Geometry: final body of the model. Coordinates: model frame, mm. A direction names the side the tool comes from. Give positions to 0.01 mm unless a question says otherwise; leave off trailing zeros. Write each loop counter-clockwise with the first axis right and the second up, starting at its lowest first coordinate (ties: lowest second). Pieces come first, ordered by that corner, then holes. Notation, with made-up numbers: (84.5, -23) -> (92.5, -23) arc R13 ccw to (92.5, 2) -> close; hole circle Ø1 at (-32.75, 33.25). An arc over 180 degrees is marked (long way). Answer in a Markdown table with one row per item. Add a question column.
Item 1: Section query B-B on y = 12. Output: boundary loops of the cut face in (x, z).
Item 2: Draft query along X for faces 1 (the flat face through (3, 18, -18)), 2 (the cylindrical face through (-8, 3, 6)). Return one class per face: +X half, -X half, draft (parallel to the pull), parting line (faces both ways), or undercut.
Item 3: Section query D-D on y = 8. Output: boundary loops of the cut face in (x, z), plus the area to 3 significant figures.
Item 4: Section query A-A on y = 4. Output: boundary loops of the cut face in (x, z).
Item 5: First-contact query: P1, Ø6, axis at x = -0.5, z = -1, coming from the -Y side; P2, Ø2, axis at x = 9, z = -13, coming from the -Y side; P3, Ø5.5, axis at y = 3, z = 1.5, coming from the +X side; P4, Ø1.5, axis at x = -10.5, z = 12, coming from the -Y side. Flat tips, straight axial feed; report the tip coordinate or a pass-through.
Item 6: Section query C-C on x = -7. State how many separate pieces and enclosed holes the cut face has, plus the area to 3 significant figures.
Item 7: Material intervals for probe 1 along X at (y, z) = (14, 0); probe 2 along Z at (x, y) = (-11.5, 3.25); probe 3 along X at (y, z) = (3.75, 12), sorted ascending. Write a range as from..to.
Item 8: Access query for faces 3 (the cylindrical face through (3.048, 2.958, 9.524)), 4 (the flat face through (-3.12, 2.46, 5.3)), 5 (the flat face through (0, 6, 3)). Directions: +Z, -Z, +X, -X, +Y, -Y. A direction counts if a zero-diameter tool reaches every point of the face in a straight line with its end or side. Return the directions, or none.
```python
from build123d import *
from build123d.topology import SkipClean

# Parameters (mm, degrees)
SKETCH1_R           = 18
BOSS_EXTRUDE1_DEPTH = 6
CUT_EXTRUDE1_DEPTH  = 5
SKETCH1_28_R        = 2.1
CUT_EXTRUDE2_DEPTH  = 27.153393661
SKETCH1_29_R        = 20
SKETCH1_29_R_2      = 18
BOSS_EXTRUDE2_DEPTH = 18
CUT_EXTRUDE3_DEPTH  = 10
BOSS_EXTRUDE3_START = -12
SKETCH1_30_R        = 20
SKETCH1_30_R_2      = 18
BOSS_EXTRUDE3_DEPTH = 12
FILLET1_ANGLE       = 36
FILLET1_2_ANGLE     = 36
FILLET1_3_ANGLE     = 36
FILLET1_4_ANGLE     = 36
FILLET1_5_ANGLE     = 36


with BuildPart() as part:
    # Sketch1 → Boss-Extrude1 (new body)
    with BuildSketch(Plane(origin=(0, 0, 0), x_dir=(1, 0, 0), z_dir=(0, 1, 0))):
        with Locations(Location((0, 0, 0), (0, 0, 270))):
            Circle(SKETCH1_R)
    extrude(amount=BOSS_EXTRUDE1_DEPTH)

    # Sketch1<27> → Cut-Extrude1 (cut)
    with BuildSketch(Plane(origin=(0, 0, 0), x_dir=(1, 0, 0), z_dir=(0, 1, 0))):
        Polygon((0, -7.101408311), (6.15, -3.550704156), (6.15, 3.550704156), (0, 7.101408311), (-6.15, 3.550704156), (-6.15, -3.550704156), align=None)
    extrude(amount=CUT_EXTRUDE1_DEPTH, mode=Mode.SUBTRACT)

    # Sketch1<28> → Cut-Extrude2 (cut, through all)
    with BuildSketch(Plane(origin=(0, 0, 0), x_dir=(1, 0, 0), z_dir=(0, 1, 0))):
        with Locations(Location((0, 0, 0), (0, 0, 270))):
            Circle(SKETCH1_28_R)
    extrude(amount=CUT_EXTRUDE2_DEPTH, mode=Mode.SUBTRACT)

    # Sketch1<29> → Boss-Extrude2 (add)
    with BuildSketch(Plane(origin=(0, 0, 0), x_dir=(1, 0, 0), z_dir=(0, 1, 0))):
        with Locations(Location((0, 0, 0), (0, 0, 270))):
            Circle(SKETCH1_29_R)
        with Locations(Location((0, 0, 0), (0, 0, 270))):
            Circle(SKETCH1_29_R_2, mode=Mode.SUBTRACT)
    extrude(amount=BOSS_EXTRUDE2_DEPTH)

    # Sketch2 → Cut-Extrude3 (cut)
    with SkipClean():  # the faces are left unmerged after this step: merging them gives an invalid solid
        with BuildSketch(Plane.XZ):
            with BuildLine():
                ThreePointArc((5.877852523, -8.090169944), (3.090169944, -9.510565163), (0, -10))
                Line((0, -10), (0, -18))
                ThreePointArc((0, -18), (5.562305899, -17.119017293), (10.580134541, -14.562305899))
                Line((10.580134541, -14.562305899), (5.877852523, -8.090169944))
            make_face()
            with BuildLine():
                Line((-10.580134541, -14.562305899), (-5.877852523, -8.090169944))
                ThreePointArc((-5.877852523, -8.090169944), (-8.090169944, -5.877852523), (-9.510565163, -3.090169944))
                Line((-9.510565163, -3.090169944), (-17.119017293, -5.562305899))
                ThreePointArc((-17.119017293, -5.562305899), (-14.562305899, -10.580134541), (-10.580134541, -14.562305899))
            make_face()
            with BuildLine():
                Line((-17.119017293, 5.562305899), (-9.510565163, 3.090169944))
                ThreePointArc((-9.510565163, 3.090169944), (-8.090169944, 5.877852523), (-5.877852523, 8.090169944))
                Line((-5.877852523, 8.090169944), (-10.580134541, 14.562305899))
                ThreePointArc((-10.580134541, 14.562305899), (-14.562305899, 10.580134541), (-17.119017293, 5.562305899))
            make_face()
            with BuildLine():
                Line((0, 18), (0, 10))
                ThreePointArc((0, 10), (3.090169944, 9.510565163), (5.877852523, 8.090169944))
                Line((5.877852523, 8.090169944), (10.580134541, 14.562305899))
                ThreePointArc((10.580134541, 14.562305899), (5.562305899, 17.119017293), (0, 18))
            make_face()
            with BuildLine():
                ThreePointArc((10, 0), (9.876883406, -1.56434465), (9.510565163, -3.090169944))
                Line((9.510565163, -3.090169944), (17.119017293, -5.562305899))
                ThreePointArc((17.119017293, -5.562305899), (17.778390131, -2.815820371), (18, 0))
                ThreePointArc((18, 0), (17.778390131, 2.815820371), (17.119017293, 5.562305899))
                Line((17.119017293, 5.562305899), (9.510565163, 3.090169944))
                ThreePointArc((9.510565163, 3.090169944), (9.876883406, 1.56434465), (10, 0))
            make_face()
        extrude(amount=-CUT_EXTRUDE3_DEPTH, mode=Mode.SUBTRACT)
    add(part.part.scale(1), mode=Mode.REPLACE)  # the faces are merged on a copy

    # Sketch1<30> → Boss-Extrude3 (add)
    with SkipClean():  # the faces are left unmerged after this step: merging them gives an invalid solid
        with BuildSketch(Plane(origin=(0, 0, 0), x_dir=(1, 0, 0), z_dir=(0, 1, 0)).offset(BOSS_EXTRUDE3_START)):
            with Locations(Location((0, 0, 0), (0, 0, 270))):
                Circle(SKETCH1_30_R)
            with Locations(Location((0, 0, 0), (0, 0, 270))):
                Circle(SKETCH1_30_R_2, mode=Mode.SUBTRACT)
        extrude(amount=BOSS_EXTRUDE3_DEPTH)

    # Fillet1: read off the stored shape, not the designer's step
    # Fillet1 outline → Fillet1 (revolve)
    with SkipClean():  # the faces are left unmerged after this step: merging them gives an invalid solid
        with BuildSketch(Plane(origin=(0, 0, 0), x_dir=(-0.9510565162951906, 0, -0.3090169943748335), z_dir=(0.3090169943748335, 0, -0.9510565162951906))):
            with BuildLine():
                ThreePointArc((18, 11), (16.535533906, 7.464466094), (13, 6))
                Line((13, 6), (18, 6))
                Line((18, 6), (18, 11))
            make_face()
            with BuildLine():
                Line((18, 0), (13, 0))
                ThreePointArc((13, 0), (16.535533906, -1.464466094), (18, -5))
                Line((18, -5), (18, 0))
            make_face()
        revolve(axis=Axis((0, 0, 0), (0, 1, 0)), revolution_arc=FILLET1_ANGLE)

    # Fillet1 2 outline → Fillet1 2 (revolve)
    with SkipClean():  # the faces are left unmerged after this step: merging them gives an invalid solid
        with BuildSketch(Plane(origin=(0, 0, 0), x_dir=(-0.5877852522922776, 0, 0.8090169943750894), z_dir=(-0.8090169943750894, 0, -0.5877852522922776))):
            with BuildLine():
                ThreePointArc((18, 11), (16.535533906, 7.464466094), (13, 6))
                Line((13, 6), (18, 6))
                Line((18, 6), (18, 11))
            make_face()
            with BuildLine():
                Line((18, 0), (13, 0))
                ThreePointArc((13, 0), (16.535533906, -1.464466094), (18, -5))
                Line((18, -5), (18, 0))
            make_face()
        revolve(axis=Axis((0, 0, 0), (0, 1, 0)), revolution_arc=FILLET1_2_ANGLE)

    # Fillet1 3 outline → Fillet1 3 (revolve)
    with SkipClean():  # the faces are left unmerged after this step: merging them gives an invalid solid
        with BuildSketch(Plane(origin=(0, 0, 0), x_dir=(0.5877852522925205, 0, 0.809016994374913), z_dir=(-0.809016994374913, 0, 0.5877852522925205))):
            with BuildLine():
                ThreePointArc((18, 11), (16.535533906, 7.464466094), (13, 6))
                Line((13, 6), (18, 6))
                Line((18, 6), (18, 11))
            make_face()
            with BuildLine():
                Line((18, 0), (13, 0))
                ThreePointArc((13, 0), (16.535533906, -1.464466094), (18, -5))
                Line((18, -5), (18, 0))
            make_face()
        revolve(axis=Axis((0, 0, 0), (0, 1, 0)), revolution_arc=FILLET1_3_ANGLE)

    # Fillet1 4 outline → Fillet1 4 (revolve)
    with SkipClean():  # the faces are left unmerged after this step: merging them gives an invalid solid
        with BuildSketch(Plane(origin=(0, 0, 0), x_dir=(0, 0, -1), z_dir=(1, 0, 0))):
            with BuildLine():
                ThreePointArc((18, 11), (16.535533906, 7.464466094), (13, 6))
                Line((13, 6), (18, 6))
                Line((18, 6), (18, 11))
            make_face()
            with BuildLine():
                Line((18, 0), (13, 0))
                ThreePointArc((13, 0), (16.535533906, -1.464466094), (18, -5))
                Line((18, -5), (18, 0))
            make_face()
        revolve(axis=Axis((0, 0, 0), (0, 1, 0)), revolution_arc=FILLET1_4_ANGLE)

    # Fillet1 5 outline → Fillet1 5 (revolve)
    with SkipClean():  # the faces are left unmerged after this step: merging them gives an invalid solid
        with BuildSketch(Plane(origin=(0, 0, 0), x_dir=(0.9510565162951443, 0, -0.3090169943749758), z_dir=(0.3090169943749758, 0, 0.9510565162951443))):
            with BuildLine():
                ThreePointArc((18, 11), (16.535533906, 7.464466094), (13, 6))
                Line((13, 6), (18, 6))
                Line((18, 6), (18, 11))
            make_face()
            with BuildLine():
                Line((18, 0), (13, 0))
                ThreePointArc((13, 0), (16.535533906, -1.464466094), (18, -5))
                Line((18, -5), (18, 0))
            make_face()
        revolve(axis=Axis((0, 0, 0), (0, 1, 0)), revolution_arc=FILLET1_5_ANGLE)


solid = part.part
```
Findings below:
| question | item | result |
|---|---|---|
| 1 | outline | circle Ø40 at (0, 0); hole circle Ø36 at (0, 0) |
| 2 | face 1 | draft |
| 2 | face 2 | undercut |
| 3 | outline | circle Ø40 at (0, 0); hole (-17.12, -5.56) arc R18 ccw to (-10.58, -14.56) -> (-9.99, -13.75) arc R17 ccw to (0, -17) -> (0, -18) arc R18 ccw to (10.58, -14.56) -> (9.99, -13.75) arc R17 ccw to (16.17, -5.25) -> (17.12, -5.56) arc R18 ccw to (17.12, 5.56) -> (16.17, 5.25) arc R17 ccw to (9.99, 13.75) -> (10.58, 14.56) arc R18 ccw to (0, 18) -> (0, 17) arc R17 ccw to (-9.99, 13.75) -> (-10.58, 14.56) arc R18 ccw to (-17.12, 5.56) -> (-16.17, 5.25) arc R17 ccw to (-16.17, -5.25) -> close |
| 3 | area | 294 mm^2 |
| 4 | outline | circle Ø40 at (0, 0); hole (-17.12, -5.56) arc R18 ccw to (-10.58, -14.56) -> (-5.88, -8.09) arc R10 cw to (-9.51, -3.09) -> close; hole (-17.12, 5.56) -> (-9.51, 3.09) arc R10 cw to (-5.88, 8.09) -> (-10.58, 14.56) arc R18 ccw to start; hole (-6.15, -3.55) -> (0, -7.1) -> (6.15, -3.55) -> (6.15, 3.55) -> (0, 7.1) -> (-6.15, 3.55) -> close; hole (0, -18) arc R18 ccw to (10.58, -14.56) -> (5.88, -8.09) arc R10 cw to (0, -10) -> close; hole (0, 10) arc R10 cw to (5.88, 8.09) -> (10.58, 14.56) arc R18 ccw to (0, 18) -> close; hole (9.51, -3.09) -> (17.12, -5.56) arc R18 ccw to (17.12, 5.56) -> (9.51, 3.09) arc R10 cw to start |
| 5 | P1 | stops at y = 5 |
| 5 | P2 | stops at y = -1.68 |
| 5 | P3 | stops at x = 20 |
| 5 | P4 | passes through |
| 6 | separate pieces | 3 |
| 6 | enclosed holes | 0 |
| 6 | area | 322 mm^2 |
| 7 | probe 1 | x = -20..-18, 18..20 |
| 7 | probe 2 | z = -16.36..-13.85, -3.74..3.74, 13.85..16.36 |
| 7 | probe 3 | x = -16..-13.42, -8.72..0, 8.72..16 |
| 8 | face 3 | +Y, -Y |
| 8 | face 4 | -Y |
| 8 | face 5 | +Y |
